from build123d import *


with BuildPart() as f1:
    # F0 (on Top) → F1 (revolve)
    with BuildSketch(Plane.XY):
        with BuildLine():
            Line((-20.1, 0), (-18.9, 0))
            Line((-18.9, 0), (-18.9, 2.25))
            Line((-18.9, 2.25), (-19.1, 2.25))
            ThreePointArc((-19.1, 2.25), (-19.807107, 1.957107), (-20.1, 1.25))
            Line((-20.1, 1.25), (-20.1, 0))
        make_face()
        with BuildLine():
            Line((-18.4, -1.75), (-18.4, 0))
            Line((-18.4, 0), (-18.9, 0))
            Line((-18.9, 0), (-18.9, -2.25))
            ThreePointArc((-18.9, -2.25), (-18.546447, -2.103553), (-18.4, -1.75))
        make_face()
        with BuildLine():
            Line((-18.9, 0), (-18.4, 0))
            Line((-18.4, 0), (-18.4, 1.75))
            ThreePointArc((-18.4, 1.75), (-18.546447, 2.103553), (-18.9, 2.25))
            Line((-18.9, 2.25), (-18.9, 0))
        make_face()
        with BuildLine():
            Line((-18.9, -2.25), (-18.9, 0))
            Line((-18.9, 0), (-20.1, 0))
            Line((-20.1, 0), (-20.1, -1.25))
            ThreePointArc((-20.1, -1.25), (-19.807107, -1.957107), (-19.1, -2.25))
            Line((-19.1, -2.25), (-18.9, -2.25))
        make_face()
    revolve(axis=Axis((0, -5.353777, 0), (0, -1, 0)))


solid = f1.part
Model file for the job. Use its own axes, mm. Coordinates: 2 decimals unless noted, no trailing zeros. Order: outer loops, then holes, each group sorted by start corner. A loop starts at its lowest first (then second) coordinate and runs counter-clockwise, first axis right, second up. Notation, with made-up numbers: (53, 38) -> (99, 38) arc R23 cw to (99, 58) -> close; hole circle Ø11 at (-5, -35.5). An arc over 180 degrees is marked (long way). Return JSON: item names as keys, results as strings. Group by question number.
Item 1: Saw through at B-B on z = 0. Write the cut outline in (x, y).
Item 2: Pull direction Z, two halves, no side cores. Call faces 1 (the cylindrical face through (14.6, 0, 11.2)), 2 (the cylindrical face through (-19.17, -0.02, -6.04)): pulls with the +Z half, pulls with the -Z half, needs draft (parallel to the pull), parting line crosses it, or undercut.
Item 3: Saw through at A-A on x = 0. Write the cut outline in (y, z), then the cut area to 3 significant figures.
Item 4: Wall check: line 1 along Z through (x, y) = (0, 0.95); line 2 along X through (y, z) = (-0.1, 17). Give the ranges that are in metal, low to high. Write a range as [from, to].
Item 5: Flat gauge pins, fed straight in: P1, Ø1, axis at y = -1, z = 2, coming from the +X side; P2, Ø1, axis at x = -5.5, y = -1.5, coming from the +Z side. Where does each tip first touch, or does it go through?
Item 6: Saw through at C-C on y = 0.25. Write the cut outline in (x, z).
Values found:
{
 "1": {"outline": "(-20.1, -1.25) arc R1 ccw to (-19.1, -2.25) -> (-18.9, -2.25) arc R0.5 ccw to (-18.4, -1.75) -> (-18.4, 1.75) arc R0.5 ccw to (-18.9, 2.25) -> (-19.1, 2.25) arc R1 ccw to (-20.1, 1.25) -> close; (18.4, -1.75) arc R0.5 ccw to (18.9, -2.25) -> (19.1, -2.25) arc R1 ccw to (20.1, -1.25) -> (20.1, 1.25) arc R1 ccw to (19.1, 2.25) -> (18.9, 2.25) arc R0.5 ccw to (18.4, 1.75) -> close"},
 "2": {"face 1": "undercut", "face 2": "parting line crosses it"},
 "3": {"outline": "(-2.25, -19.1) arc R1 ccw to (-1.25, -20.1) -> (1.25, -20.1) arc R1 ccw to (2.25, -19.1) -> (2.25, -18.9) arc R0.5 ccw to (1.75, -18.4) -> (-1.75, -18.4) arc R0.5 ccw to (-2.25, -18.9) -> close; (-2.25, 18.9) arc R0.5 ccw to (-1.75, 18.4) -> (1.75, 18.4) arc R0.5 ccw to (2.25, 18.9) -> (2.25, 19.1) arc R1 ccw to (1.25, 20.1) -> (-1.25, 20.1) arc R1 ccw to (-2.25, 19.1) -> close", "area": "14.2 mm2"},
 "4": {"line 1": "z = [-20.1, -18.4], [18.4, 20.1]", "line 2": "x = [-10.72, -7.04], [7.04, 10.72]"},
 "5": {"P1": "stops at x = 20.04", "P2": "stops at z = 19.46"},
 "6": {"outline": "circle Ø40.2 at (0, 0); hole circle Ø36.8 at (0, 0)"}
}
